Can you work these out from the model? Positions are in its coordinate system, mm. Give positions to 0.01 mm unless a question says otherwise; leave off trailing zeros. Order: outer loops, then holes, each group sorted by start corner. A loop starts at its lowest first (then second) coordinate and runs counter-clockwise, first axis right, second up. Notation, with made-up numbers: (88, -10) - (116, -10) arc R22 ccw to (116, 19) - close; hole circle Ø6 at (0, -1). An arc over 180 degrees is marked (long way). Answer as a JSON object with one key per item and string values.
```python
from build123d import *

# Parameters (mm, degrees)
SKETCH1_R           = 25
SKETCH1_R_2         = 20
BOSS_EXTRUDE1_DEPTH = 2
SKETCH2_R           = 25
BOSS_EXTRUDE2_DEPTH = 1
SKETCH3_R           = 20
CUT_EXTRUDE1_DEPTH  = 1


with BuildPart() as part:
    # Sketch1 → Boss-Extrude1 (new body)
    with BuildSketch(Plane.XY):
        Circle(SKETCH1_R)
        Circle(SKETCH1_R_2, mode=Mode.SUBTRACT)
    extrude(amount=BOSS_EXTRUDE1_DEPTH)

    # Sketch2 → Boss-Extrude2 (add)
    with BuildSketch(Plane.XY.offset(2)):
        Circle(SKETCH2_R)
    extrude(amount=BOSS_EXTRUDE2_DEPTH)

    # Sketch3 → Cut-Extrude1 (cut)
    with BuildSketch(Plane(origin=(0, 0, 2), x_dir=(-1, 0, 0), z_dir=(0, 0, -1))):
        Circle(SKETCH3_R)
    extrude(amount=-CUT_EXTRUDE1_DEPTH, mode=Mode.SUBTRACT)


solid = part.part
```
Q1. I'm going to push a flat-ended pin straight in: pin 1 Ø1 at (y, z) = (19.5, 0.5) entering from +X. Where does the tip first touch, or does it pass through?
Recorded:
{"pin 1": "stops at x = 16.25"}
Q2. If we section it at A-A, the plane y = 0: Please give me the cut outline in (x, z).
Recorded:
{"outline": "(-25, 0) - (-20, 0) - (-20, 3) - (-25, 3) - close; (20, 0) - (25, 0) - (25, 3) - (20, 3) - close"}
Q3. If we section it at C-C, the plane z = 1.3: Please give me the cut outline in (x, y), then the cut area to 3 significant figures.
Recorded:
{"outline": "circle Ø50 at (0, 0); hole circle Ø40 at (0, 0)", "area": "707 mm^2"}
Q4. I need wall thicknesses on L1, parallel to Y at x = 0, z = 1.05; L2, parallel to Y at x = 3, z = 2.2; L3, parallel to X at y = 10, z = 1. Which ranges of each line are inside material? Lowest first, please.
Recorded:
{"L1": "y = -25 to -20, 20 to 25", "L2": "y = -24.82 to -19.77, 19.77 to 24.82", "L3": "x = -22.91 to -17.32, 17.32 to 22.91"}
